from build123d import *

# Parameters (mm, degrees)
BOSS_EXTRUDE1_DEPTH = 1.6
SKETCH2_W           = 9.9
SKETCH2_H           = 6.5
BOSS_EXTRUDE2_DEPTH = 5.7
SKETCH3_W           = 8.4
SKETCH3_H           = 4.2
CUT_EXTRUDE1_DEPTH  = 5.75
SKETCH4_R           = 1.75
CUT_EXTRUDE2_DEPTH  = 5.75
SKETCH5_W           = 12.7
SKETCH5_H           = 6.1
BOSS_EXTRUDE3_DEPTH = 5.75
BOSS_EXTRUDE4_DEPTH = 5.75
SKETCH8_W           = 1.45
SKETCH8_H           = 1.30003701
CUT_EXTRUDE3_DEPTH  = 10


with BuildPart() as part:
    # Sketch1 → Boss-Extrude1 (new body)
    with BuildSketch(Plane.XY):
        with BuildLine():
            Line((0, -6.9), (0, -13))
            Line((0, -13), (13, -13))
            Line((13, -13), (13, -6.9))
            Line((13, -6.9), (16.5, -6.9))
            ThreePointArc((16.5, -6.9), (19.95, -3.45), (16.5, 0))
            Line((16.5, 0), (13, 0))
            Line((13, 0), (0, 0))
            Line((0, 0), (-3.5, 0))
            ThreePointArc((-3.5, 0), (-6.95, -3.45), (-3.5, -6.9))
            Line((-3.5, -6.9), (0, -6.9))
        make_face()
    extrude(amount=BOSS_EXTRUDE1_DEPTH)

    # Sketch2 → Boss-Extrude2 (add)
    with BuildSketch(Plane.XY.offset(1.6)):
        with Locations((6.5, -14.25)):
            Rectangle(SKETCH2_W, SKETCH2_H)
    extrude(amount=BOSS_EXTRUDE2_DEPTH)

    # Sketch3 → Cut-Extrude1 (cut)
    with BuildSketch(Plane.XZ.offset(17.5)):
        with Locations((6.5, 4.45)):
            Rectangle(SKETCH3_W, SKETCH3_H)
    extrude(amount=-CUT_EXTRUDE1_DEPTH, mode=Mode.SUBTRACT)

    # Sketch4 → Cut-Extrude2 (cut)
    with BuildSketch(Plane.XY.offset(1.6)):
        with Locations((-3.5, -3.45)):
            Circle(SKETCH4_R)
        with Locations((16.5, -3.45)):
            Circle(SKETCH4_R)
    extrude(amount=-CUT_EXTRUDE2_DEPTH, mode=Mode.SUBTRACT)

    # Sketch5 → Boss-Extrude3 (add)
    with BuildSketch(Plane.XY.offset(1.6)):
        with Locations((6.5, 1.95)):
            Rectangle(SKETCH5_W, SKETCH5_H)
    extrude(amount=BOSS_EXTRUDE3_DEPTH)

    # Sketch7 → Boss-Extrude4 (add)
    with BuildSketch(Plane.XY.offset(7.35)):
        with BuildLine():
            Line((3.9, 5), (3.9, 5.838508632))
            ThreePointArc((3.9, 5.838508632), (4.061491368, 6), (4.222982736, 5.838508632))
            Line((4.222982736, 5.838508632), (4.222982736, 5))
            Line((4.222982736, 5), (3.9, 5))
        make_face()
    extrude(amount=-BOSS_EXTRUDE4_DEPTH)

    # Sketch8 → Cut-Extrude3 (cut)
    with BuildSketch(Plane(origin=(12.85, 0, 0), x_dir=(0, 0, -1), z_dir=(1, 0, 0))):
        with Locations((-6.625, 5.650018505)):
            Rectangle(SKETCH8_W, SKETCH8_H)
        with Locations((-2.325, 5.650018505)):
            Rectangle(SKETCH8_W, SKETCH8_H)
    extrude(amount=-CUT_EXTRUDE3_DEPTH, mode=Mode.SUBTRACT)


solid = part.part
Geometry check sheet. Reference: the model listing, model coordinates, mm. A direction names the side the tool comes from. Round coordinates to 2 decimals unless told otherwise and drop trailing zeros. Loops run counter-clockwise (first coordinate to the right, second up) from the corner with the lowest first, then second, coordinate; pieces in that order, holes last.
Item 1: Mould release check, pull along X, two halves, no side actions. Record for faces 1 (the flat face through (6, -11, 4)), 2 (the flat face through (2.3, -15, 4)), 3 (the flat face through (0.15, 2, 4)): pulls with the +X half, pulls with the -X half, needs draft (parallel to the pull), parting line crosses it, or undercut.
Item 2: Gauge pin test, flat ends, axial feed: pin 1 (3 mm diameter, centred on y = 1.5, z = 5, fed in from -X); pin 2 (1.3 mm diameter, centred on y = -11.5, z = 1, fed in from +X); pin 3 (4.5 mm diameter, centred on x = 6.5, y = -14.5, fed in from +Z). Record the tip position at first contact, or that the pin passes through.
Item 3: Access from +Z, -Z, +X, -X, +Y, -Y to the whole of each face (thin tool, end or side, straight path). Record for faces 4 (the flat face through (6, -13, 1)), 5 (the flat face through (13, -10, 1)), 6 (the flat face through (1.55, -14, 4)), 7 (the flat face through (4.223, 5.4, 4.5)).
Item 4: Cross-section at D-D on z = 4.75. Record the boundary of the cut face in (x, y).
Item 5: Cross-section at A-A on z = 2. Record the boundary of the cut face in (x, y).
Item 6: Cross-section at B-B on y = -12.5. Record the boundary of the cut face in (x, z).
Item 7: Cross-section at C-C on y = -3.45. Record the boundary of the cut face in (x, z), then the cut area to 3 significant figures.
Item 8: Thickness scan on line 1 (X direction, y = -14.25, z = 3.5); line 2 (Y direction, x = 4.75, z = 4.75); line 3 (Y direction, x = -3.5, z = 0.4). Record the ranges inside material, lowest first.
Answer sheet:
1. face 1: needs draft
1. face 2: undercut
1. face 3: pulls with the -X half
2. pin 1: stops at x = 0.15
2. pin 2: stops at x = 13
2. pin 3: stops at z = 7.3
3. face 4: -Z, +X, -X, -Y
3. face 5: +Z, -Z, +X, -Y
3. face 6: +Z, -X, -Y
3. face 7: +Z, -Z, +X, +Y
4. outline: (0.15, -1.1) - (12.85, -1.1) - (12.85, 5) - (4.22, 5) - (4.22, 5.84) arc R0.16 ccw to (3.9, 5.84) - (3.9, 5) - (0.15, 5) - close; (1.55, -17.5) - (2.3, -17.5) - (2.3, -11.75) - (10.7, -11.75) - (10.7, -17.5) - (11.45, -17.5) - (11.45, -11) - (1.55, -11) - close
5. outline: (0.15, -1.1) - (12.85, -1.1) - (12.85, 5) - (0.15, 5) - close; (1.55, -17.5) - (11.45, -17.5) - (11.45, -11) - (1.55, -11) - close
6. outline: (0, 0) - (13, 0) - (13, 1.6) - (11.45, 1.6) - (11.45, 7.3) - (1.55, 7.3) - (1.55, 1.6) - (0, 1.6) - close; hole (2.3, 2.35) - (10.7, 2.35) - (10.7, 6.55) - (2.3, 6.55) - close
7. outline: (-6.95, 0) - (-5.25, 0) - (-5.25, 1.6) - (-6.95, 1.6) - close; (-1.75, 0) - (14.75, 0) - (14.75, 1.6) - (-1.75, 1.6) - close; (18.25, 0) - (19.95, 0) - (19.95, 1.6) - (18.25, 1.6) - close
7. area: 31.8 mm2
8. line 1: x = 1.55 to 2.3, 10.7 to 11.45
8. line 2: y = -11.75 to -11, -1.1 to 5
8. line 3: y = -6.9 to -5.2, -1.7 to 0
